from build123d import *

# Parameters (mm, degrees)
CROQUIS1_R              = 5
SALIENTE_EXTRUIR1_DEPTH = 108
CROQUIS2_R              = 2.5
CORTAR_EXTRUIR1_DEPTH   = 10


with BuildPart() as part:
    # Croquis1 → Saliente-Extruir1 (new body)
    with BuildSketch(Plane(origin=(0, 0, 0), x_dir=(1, 0, 0), z_dir=(0, 1, 0))):
        with Locations(Location((0, 0, 0), (0, 0, 270))):
            Circle(CROQUIS1_R)
    extrude(amount=SALIENTE_EXTRUIR1_DEPTH)

    # Croquis2 → Cortar-Extruir1 (cut)
    with BuildSketch(Plane.XZ):
        with Locations(Location((0, 0, 0), (0, 0, 270))):
            Circle(CROQUIS2_R)
    cortar_extruir1 = extrude(amount=-CORTAR_EXTRUIR1_DEPTH, mode=Mode.SUBTRACT)

    # Simetría1: Cortar-Extruir1 across plane
    add(cortar_extruir1.mirror(Plane(origin=(0, 54, 0), x_dir=(0, 0, 1), z_dir=(0, -1, 0))), mode=Mode.SUBTRACT)


solid = part.part
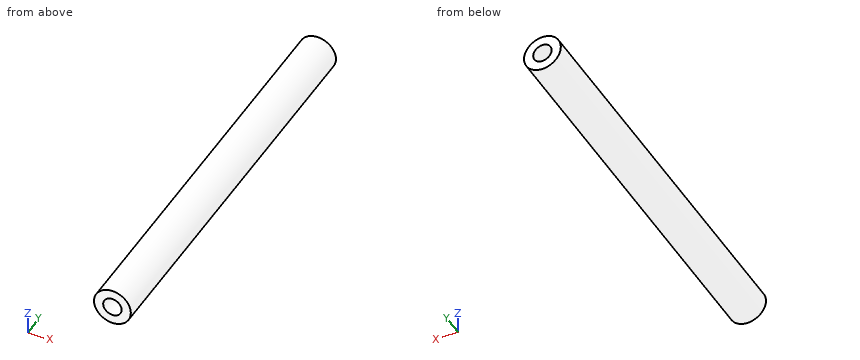
Source: CAD feature listing. Evaluate the final solid. Frame: model axes, mm. Give positions to 0.01 mm unless a question says otherwise; leave off trailing zeros. Write each loop counter-clockwise with the first axis right and the second up, starting at its lowest first coordinate (ties: lowest second). Pieces come first, ordered by that corner, then holes. Notation, with made-up numbers: (52, -8.5) -> (81, -8.5) arc R21 ccw to (81, 22.5) -> close; hole circle Ø11 at (37, 75). An arc over 180 degrees is marked (long way). Return JSON: item names as keys, results as strings. Group by question number.
1. Section B-B, the plane z = 0. Output: boundary loops of the cut face in (x, y).
2. Section A-A, the plane x = 0. Output: boundary loops of the cut face in (y, z).
3. Material intervals for line 1 (X direction, y = 105, z = 0); line 2 (X direction, y = 74, z = -0.25); line 3 (X direction, y = 99.5, z = 1.5), sorted ascending. Write a range as from..to.
4. Pin query (flat end, axial travel): pin 1 Ø5 at (x, z) = (0.5, -3.5) entering from -Y; pin 2 Ø4.5 at (x, z) = (0, 0) entering from +Y; pin 3 Ø2.5 at (x, z) = (1, -0.5) entering from -Y. Return the tip coordinate at first contact, or that it passes through.
5. Section C-C, the plane y = 93. Output: boundary loops of the cut face in (x, z), then the cut area to 3 significant figures.
Determined:
{
 "1": {"outline": "(-5, 0) -> (-2.5, 0) -> (-2.5, 10) -> (2.5, 10) -> (2.5, 0) -> (5, 0) -> (5, 108) -> (2.5, 108) -> (2.5, 98) -> (-2.5, 98) -> (-2.5, 108) -> (-5, 108) -> close"},
 "2": {"outline": "(0, -5) -> (108, -5) -> (108, -2.5) -> (98, -2.5) -> (98, 2.5) -> (108, 2.5) -> (108, 5) -> (0, 5) -> (0, 2.5) -> (10, 2.5) -> (10, -2.5) -> (0, -2.5) -> close"},
 "3": {"line 1": "x = -5..-2.5, 2.5..5", "line 2": "x = -4.99..4.99", "line 3": "x = -4.77..-2, 2..4.77"},
 "4": {"pin 1": "stops at y = 0", "pin 2": "stops at y = 98", "pin 3": "stops at y = 10"},
 "5": {"outline": "circle Ø10 at (0, 0)", "area": "78.5 mm2"}
}
